Input: part model. Units: mm. Frame: model coordinates. Face numbers are marked on the shaded views. A direction names the side the tool comes from. Give positions to 0.01 mm unless a question says otherwise; leave off trailing zeros. Loops run counter-clockwise (first coordinate to the right, second up) from the corner with the lowest first, then second, coordinate; pieces in that order, holes last.
from build123d import *

# Parameters (mm, degrees)
F1_DEPTH = 25.4
F0_W     = 73.2126906514
F0_H     = 27.755683288
F2_DEPTH = 50.546
F4_DEPTH = 26.67
F5_W     = 25.4
F5_H     = 33.8419238105
F6_DEPTH = 15.24
F7_W     = 7.62
F7_H     = 20.0272031784
F8_DEPTH = 27.756683288


with BuildPart() as f1:
    # F0 (on Front) → F1 (new body)
    with BuildSketch(Plane.XZ):
        with BuildLine():
            Line((-54.8033118248, 55.7945854962), (-73.2126906514, 55.7945854962))
            Line((-73.2126906514, 55.7945854962), (-73.2126906514, -21.2415922433))
            Line((-73.2126906514, -21.2415922433), (0, -21.2415922433))
            Line((0, -21.2415922433), (0, 55.7945854962))
            Line((0, 55.7945854962), (-18.4093788266, 55.7945854962))
            Line((-18.4093788266, 55.7945854962), (-18.4093788266, 0))
            ThreePointArc((-18.4093788266, 0), (-36.6063453257, -13.5848598971), (-54.8033118248, 0))
            Line((-54.8033118248, 0), (-54.8033118248, 55.7945854962))
        make_face()
    extrude(amount=F1_DEPTH)

    # F0 (on Front) → F2 (join)
    with BuildSketch(Plane.XZ):
        with Locations((-36.6063453257, -35.1194338873)):
            Rectangle(F0_W, F0_H)
    extrude(amount=F2_DEPTH)

    # F3 (on face) → F4 (join)
    with BuildSketch(Plane.XY.offset(-21.2415922433)):
        with BuildLine():
            Line((0, -50.546), (-73.2126906514, -50.546))
            ThreePointArc((-73.2126906514, -50.546), (-36.6063453257, -87.1523453257), (0, -50.546))
        make_face()
    extrude(amount=-F4_DEPTH)

    # F5 (on face) → F6 (cut)
    with BuildSketch(Plane.YZ):
        with Locations((-12.7, -32.076313626)):
            Rectangle(F5_W, F5_H)
    extrude(amount=-F6_DEPTH, mode=Mode.SUBTRACT)

    # F7 (on face) → F8 (cut, through all)
    with BuildSketch(Plane.XY.offset(-21.2415922433)):
        with Locations((-3.81, -35.4136015892)):
            Rectangle(F7_W, F7_H)
    extrude(amount=-F8_DEPTH, mode=Mode.SUBTRACT)


solid = f1.part
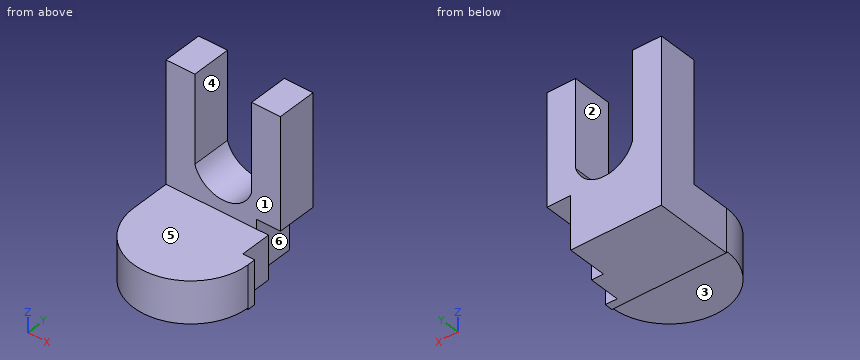
(1) Cut plane C-C (x = -4). Return the cut outline in (y, z), and give its area (3 significant figures).
Values follow:
outline: (-67.18, -47.91) - (-50.55, -47.91) - (-50.55, -49) - (-45.43, -49) - (-45.43, -21.24) - (-67.18, -21.24) - close; (-25.4, -15.16) - (0, -15.16) - (0, 55.79) - (-25.4, 55.79) - close
area: 2,390 mm2
(2) Ray query, probe 1 along X at (y, z) = (-13.5, 50.5); probe 2 along Y at (x, z) = (-59, 38); probe 3 along Z at (x, y) = (-33, -70). Return the intervals inside material, ascending.
Values follow:
probe 1: x = -73.21 to -54.8, -18.41 to 0
probe 2: y = -25.4 to 0
probe 3: z = -47.91 to -21.24
(3) Mould query, pull axis X, two halves, no side actions, for the marked faces 4, 5 and 6. Classes: +X half, -X half, draft (parallel to the pull), parting line (faces both ways), or undercut.
Values follow:
face 4: undercut
face 5: draft
face 6: +X half
(4) Cut plane A-A (z = 20.5). Return the cut outline in (x, y).
Values follow:
outline: (-73.21, -25.4) - (-54.8, -25.4) - (-54.8, 0) - (-73.21, 0) - close; (-18.41, -25.4) - (0, -25.4) - (0, 0) - (-18.41, 0) - close
(5) Reachability of the marked faces 1, 2 and 3 from +Z, -Z, +X, -X, +Y, -Y: full face, straight path, thin tool, end or side. Return the list, or none.
Values follow:
face 1: +Z, +X, -X, -Y
face 2: +Z, +Y, -Y
face 3: -Z, +X, -X, -Y
(6) Cut plane D-D (y = -15). Return the cut outline in (x, z).
Values follow:
outline: (-73.21, -49) - (-15.24, -49) - (-15.24, -15.16) - (0, -15.16) - (0, 55.79) - (-18.41, 55.79) - (-18.41, 0) arc R18.98 cw to (-54.8, 0) - (-54.8, 55.79) - (-73.21, 55.79) - close
(7) Pin query (flat end, axial travel): pin 1 Ø4 at (x, z) = (-5, -33) entering from +Y; pin 2 Ø20.5 at (y, z) = (-6.5, -29.5) entering from +X; pin 3 Ø10 at (x, y) = (-44, -23.5) entering from +Z. Return the tip coordinate at first contact, or that it passes through.
Values follow:
pin 1: stops at y = -45.43
pin 2: stops at x = -15.24
pin 3: stops at z = -8.98
